Design review of the part built by this model. Coordinates are the model's own, in mm. Face numbers are marked on the shaded views. A direction names the side the tool comes from. Give positions to 0.01 mm unless a question says otherwise; leave off trailing zeros. Write each loop counter-clockwise with the first axis right and the second up, starting at its lowest first coordinate (ties: lowest second). Pieces come first, ordered by that corner, then holes. Notation, with made-up numbers: (20, 28.25) -> (35, 28.25) arc R14 ccw to (35, 48.25) -> close; hole circle Ø11 at (-16.75, -30.5). An arc over 180 degrees is marked (long way). Answer as a JSON object with one key per item and string values.
```python
from build123d import *

# Parameters (mm, degrees)
BOSS_EXTRUDE1_DEPTH = 543.5
SKETCH4_R           = 3.96875
CUT_EXTRUDE1_DEPTH  = 559.140887232


with BuildPart() as part:
    # Sketch1 → Boss-Extrude1 (new body)
    with BuildSketch(Plane.XY):
        Polygon((0, 76.2), (0, 0), (101.6, 0), (101.6, 6.35), (6.35, 6.35), (6.35, 76.2), align=None)
    extrude(amount=BOSS_EXTRUDE1_DEPTH)

    # Sketch4 → Cut-Extrude1 (cut, through all)
    with BuildSketch(Plane.XZ):
        with Locations(Location((88.9, 530.8, 0), (0, 0, 270))):
            Circle(SKETCH4_R)
        with Locations(Location((19.05, 530.8, 0), (0, 0, 270))):
            Circle(SKETCH4_R)
        with Locations(Location((19.05, 12.7, 0), (0, 0, 270))):
            Circle(SKETCH4_R)
        with Locations(Location((88.9, 12.7, 0), (0, 0, 270))):
            Circle(SKETCH4_R)
    extrude(amount=-CUT_EXTRUDE1_DEPTH, mode=Mode.SUBTRACT)


solid = part.part
```
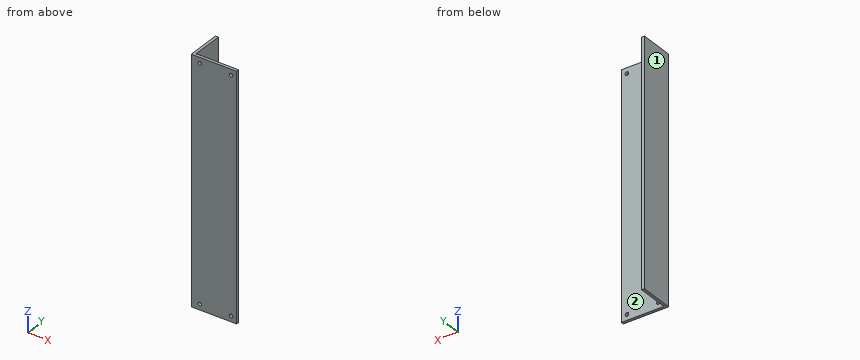
(1) We need section A-A, the plane z = 148.5. State the section outline as (x, y) points, then the cut area to 3 significant figures.
Here are the results:
{"outline": "(0, 0) -> (101.6, 0) -> (101.6, 6.35) -> (6.35, 6.35) -> (6.35, 76.2) -> (0, 76.2) -> close", "area": "1,090 mm²"}
(2) Clearance check with flat-ended pins moving along their axes: pin 1 (2 mm diameter, centred on x = 55.5, z = 401.5, fed in from +Y); pin 2 (12 mm diameter, centred on y = 66, z = 376, fed in from +X); pin 3 (7 mm diameter, centred on x = 88.9, z = 530.8, fed in from -Y). State where each tip first meets the part, or that it passes through.
Here are the results:
{"pin 1": "stops at y = 6.35", "pin 2": "stops at x = 6.35", "pin 3": "passes through"}
(3) We need section B-B, the plane x = 59. State the section outline as (y, z) points.
Here are the results:
{"outline": "(0, 0) -> (6.35, 0) -> (6.35, 543.5) -> (0, 543.5) -> close"}
(4) For the marked faces 1 and 2, list the 3-axis set-ups (+Z, -Z, +X, -X, +Y, -Y) from which the entire face can be reached by the end or side of a thin tool; tool diameter is ignored.
Here are the results:
{"face 1": "+Z, -Z, -X, +Y, -Y", "face 2": "+Z, -Z, +X, +Y"}
(5) For line 1 along X through (y, z) = (2.5, 530.8); line 2 along Z through (x, y) = (88, 1); line 3 along Z through (x, y) = (19, 5), list the stretches that pass through material, from the lowest coordinate up.
Here are the results:
{"line 1": "x = 0 to 15.08, 23.02 to 84.93, 92.87 to 101.6", "line 2": "z = 0 to 8.83, 16.57 to 526.93, 534.67 to 543.5", "line 3": "z = 0 to 8.73, 16.67 to 526.83, 534.77 to 543.5"}
